Print and shaded views of the part. All mm, measured from the part's lowest x, y and z. A direction names the side the tool comes from. Coordinates: 2 decimals unless noted, no trailing zeros. Order: outer loops, then holes, each group sorted by start corner. A loop starts at its lowest first (then second) coordinate and runs counter-clockwise, first axis right, second up.
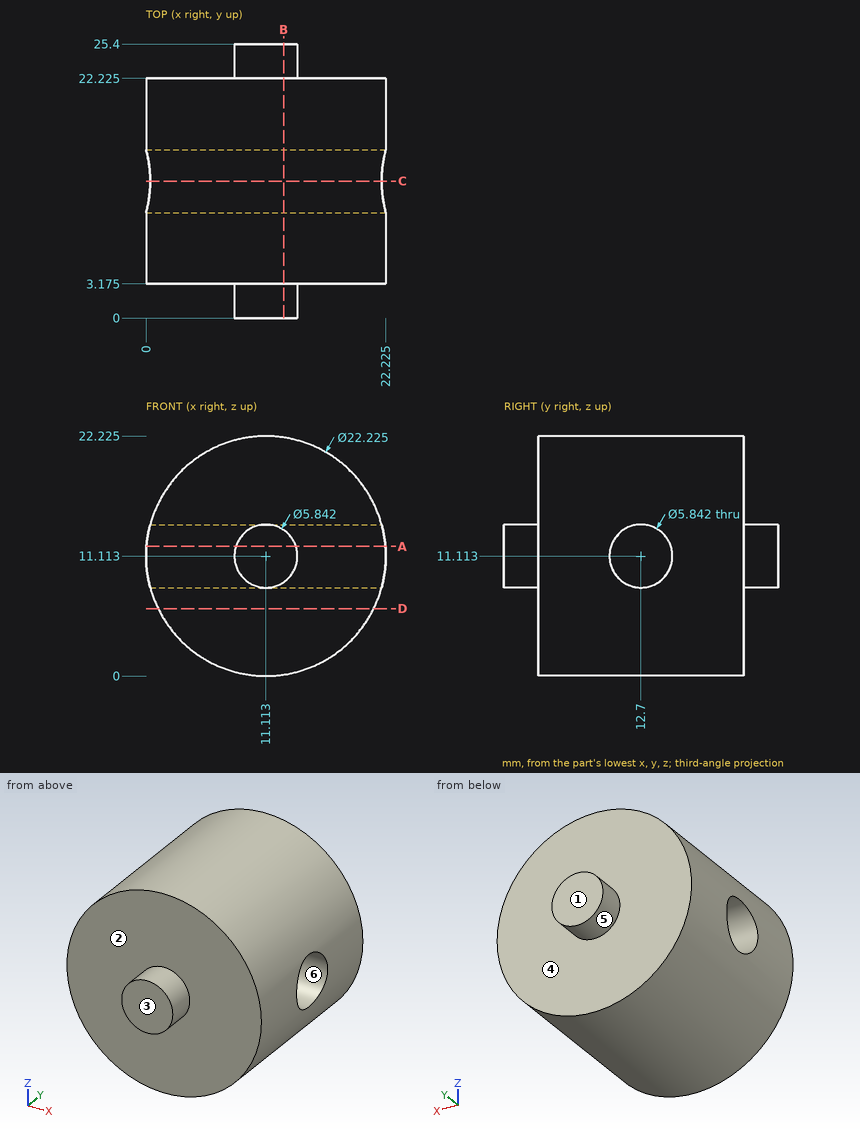
Q1. Cut at C-C, the plane y = 12.7. List the corners of the cut face in (x, z) (1 decimal), plus the area to 3 significant figures.
Established:
outline: (0.4, 8.2) arc R11.1 ccw to (21.8, 8.2) - close; (0.4, 14) - (21.8, 14) arc R11.1 ccw to start
area: 260 mm2
Q2. Mould opens along Y. For the marked faces 3, 4, 5 and 6 say: pulls with the +Y half, pulls with the -Y half, needs draft (parallel to the pull), parting line crosses it, or undercut.
Established:
face 3: pulls with the -Y half
face 4: pulls with the +Y half
face 5: needs draft
face 6: undercut
Q3. Drop flat-ended pins along their axis: P1, Ø3, axis at x = 8.5, z = 2.5, coming from the +Y side (1 decimal); P2, Ø1.5, axis at x = 7.5, y = 12.5, coming from the +Z side; P3, Ø2, axis at x = 19.5, z = 16, coming from the -Y side (1 decimal). Give the stop position or say it passes through.
Established:
P1: stops at y = 22.2
P2: stops at z = 21.85
P3: stops at y = 3.2
Q4. Which spindle directions (+Z, -Z, +X, -X, +Y, -Y) get a long thin tool onto all of the face, cutting with end or side? Do the marked faces 1 and 2. Say none if no direction does.
Established:
face 1: +Z, -Z, +X, -X, +Y
face 2: -Y
Q5. Probe line 1 (Y direction, x = 4, z = 9.5) (1 decimal); line 2 (Z direction, x = 1.75, y = 14) (1 decimal); line 3 (Z direction, x = 5, y = 14.75) (1 decimal). List the from-to ranges inside material, lowest first.
Established:
line 1: y = 3.2 to 10.3, 15.1 to 22.2
line 2: z = 5.1 to 8.5, 13.7 to 17.1
line 3: z = 1.8 to 9, 13.2 to 20.4
Q6. Cut at A-A, the plane z = 12. List the corners of the cut face in (x, y) (1 decimal), plus the area to 3 significant figures.
Established:
outline: (0, 3.2) - (8.3, 3.2) - (8.3, 0) - (13.9, 0) - (13.9, 3.2) - (22.2, 3.2) - (22.2, 9.9) - (0, 9.9) - close; (0, 15.5) - (22.2, 15.5) - (22.2, 22.2) - (13.9, 22.2) - (13.9, 25.4) - (8.3, 25.4) - (8.3, 22.2) - (0, 22.2) - close
area: 334 mm2
Q7. Cut at D-D, the plane z = 6.25. List the corners of the cut face in (x, y) (1 decimal), plus the area to 3 significant figures.
Established:
outline: (1.1, 3.2) - (21.1, 3.2) - (21.1, 22.2) - (1.1, 22.2) - close
area: 381 mm2
Q8. Cut at B-B, the plane x = 12.75. List the corners of the cut face in (y, z) (1 decimal), plus the area to 3 significant figures.
Established:
outline: (0, 8.7) - (3.2, 8.7) - (3.2, 0.1) - (22.2, 0.1) - (22.2, 8.7) - (25.4, 8.7) - (25.4, 13.5) - (22.2, 13.5) - (22.2, 22.1) - (3.2, 22.1) - (3.2, 13.5) - (0, 13.5) - close; hole circle Ø5.8 at (12.7, 11.1)
area: 423 mm2
